Geometry: final body of the model. Coordinates: model frame, mm. A direction names the side the tool comes from. Round coordinates to 2 decimals unless told otherwise and drop trailing zeros. Loops run counter-clockwise (first coordinate to the right, second up) from the corner with the lowest first, then second, coordinate; pieces in that order, holes last. Notation, with made-up numbers: (5.25, 42.5) - (19.25, 42.5) arc R27 ccw to (19.25, 62.5) - close; hole circle Ø7 at (67.5, 41). An arc over 180 degrees is marked (long way). Write item = value, one per line. Start each with the question number.
Item 1: Line query: line 1 (Y direction, x = 61, z = 34.5); line 2 (X direction, y = 20, z = 3.5); line 3 (Z direction, x = 30, y = 45.5). Output: solid intervals per line, ascending. Write a range as from..to.
Item 2: First-contact query: pin 1 (4 mm diameter, centred on x = 22, z = 25.5, fed in from +Y); pin 2 (12 mm diameter, centred on x = 25.5, y = 37, fed in from +Z); pin 3 (12 mm diameter, centred on x = 79, z = -9.5, fed in from -Y). Flat tips, straight axial feed; report the tip coordinate or a pass-through.
Item 3: Access query for faces 1 (the flat face through (20, 20, 25)), 2 (the flat face through (40, 64, 1)), 3 (the flat face through (80, 50, 1)), 4 (the flat face through (50, 40, 40)), 5 (the flat face through (24, 36, -10)). Directions: +Z, -Z, +X, -X, +Y, -Y. A direction counts if a zero-diameter tool reaches every point of the face in a straight line with its end or side. Return the directions, or none.
Item 4: Section B-B (y = 37.5). Return loops of the section in (x, z).
Item 5: Section D-D (y = 68.5). Return loops of the section in (x, z).
Item 6: Section C-C (x = 87.5). Return loops of the section in (y, z), plus the area to 3 significant figures.
Item 7: Section A-A (z = 4). Return loops of the section in (x, y), plus the area to 3 significant figures.
from build123d import *

# Parameters (mm, degrees)
BOSS_EXTRUDE1_DEPTH = 40
BOSS_EXTRUDE2_DEPTH = 10


with BuildPart() as part:
    # Sketch1 → Boss-Extrude1 (new, symmetric)
    with BuildSketch(Plane.XY):
        Polygon((40, 20), (0, 20), (0, 0), (60, 0), (60, 50), (100, 50), (100, 80), (40, 80), align=None)
    extrude(amount=BOSS_EXTRUDE1_DEPTH, both=True)

    # Sketch1_3 → Boss-Extrude2 (add, symmetric)
    with BuildSketch(Plane.XY):
        Polygon((0, 30), (0, 20), (40, 20), (40, 60), align=None)
    extrude(amount=BOSS_EXTRUDE2_DEPTH, both=True)


solid = part.part
Taken from the geometry:
q1.line_1 = 50..80
q1.line_2 = 0..60
q1.line_3 = -10..10
q2.pin_1 = 20
q2.pin_2 = 10
q2.pin_3 = 50
q3.face_1 = +Z, -X, +Y
q3.face_2 = -X, +Y
q3.face_3 = +Z, -Z, +X, -Y
q3.face_4 = +Z, +X, -X, +Y, -Y
q3.face_5 = -Z, -X, +Y
q4.outline = (10, -10) - (40, -10) - (40, -40) - (60, -40) - (60, 40) - (40, 40) - (40, 10) - (10, 10) - close
q5.outline = (40, -40) - (100, -40) - (100, 40) - (40, 40) - close
q6.outline = (50, -40) - (80, -40) - (80, 40) - (50, 40) - close
q6.area = 2,400 mm^2
q7.outline = (0, 0) - (60, 0) - (60, 50) - (100, 50) - (100, 80) - (40, 80) - (40, 60) - (0, 30) - close
q7.area = 4,600 mm^2
